The figure shows three views and two pictorial views of one solid part (mm, origin at its lowest corner). Answer the questions. Coordinates: 2 decimals unless noted, no trailing zeros. Order: outer loops, then holes, each group sorted by start corner. A loop starts at its lowest first (then second) coordinate and runs counter-clockwise, first axis right, second up. Notation, with made-up numbers: (-30, 33) -> (15, 33) arc R14 ccw to (15, 54) -> close; hole circle Ø2 at (65, 24.25). An arc over 180 degrees is marked (long way). Write item = value, one per line. Start each with the question number.
Q1. Straight lines are drawn through the part: L1, parallel to X at y = 309.5, z = 9.25; L2, parallel to Y at x = 487.5, z = 4; L3, parallel to X at y = 117, z = 6.5. For each, find the intervals that lie inside material, in ascending order. Write a range as from..to.
Q2. The part is cut by section D-D, the plane z = 14.75. Count the separate pieces of the cut face and the enclosed holes in it, plus the area to 3 significant figures.
Q3. The part is cut by section B-B, the plane y = 304.8. Determine the outline of the cut face in (x, z), plus the area to 3 significant figures.
Q4. A flat-ended cylindrical pin translates along its axis: pin 1 (5.5 mm diameter, centred on y = 216.5, z = 10.5, fed in from +X). Find the tip coordinate at first contact, or state that the pin passes through.
Q5. The part is cut by section A-A, the plane x = 44.45. Determine the outline of the cut face in (y, z).
Q6. For a pull along Z with two mould halves and no side action, classify the marked faces 1 and 2 as +Z half, -Z half, draft (parallel to the pull), parting line (faces both ways), or undercut.
Q7. The part is cut by section C-C, the plane x = 469. Determine the outline of the cut face in (y, z), plus the area to 3 significant figures.
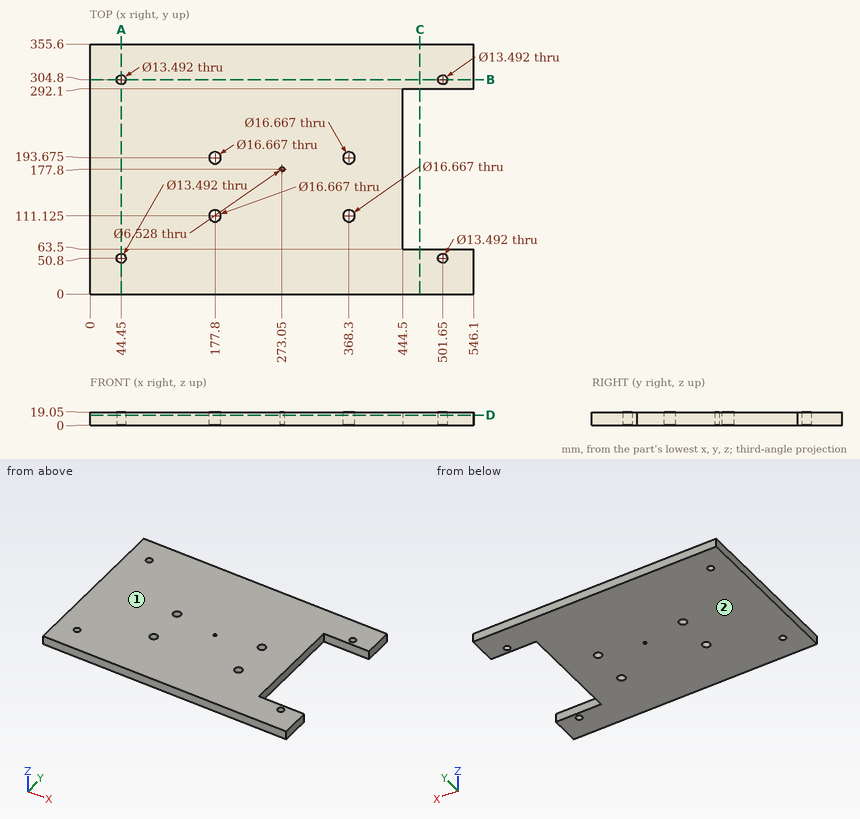
Model answer:
q1.L1 = 0..39.61, 49.29..496.81, 506.49..546.1
q1.L2 = 0..63.5, 292.1..355.6
q1.L3 = 0..171.89, 183.71..362.39, 374.21..444.5
q2.separate_pieces = 1
q2.enclosed_holes = 9
q2.area = 169,000 mm2
q3.outline = (0, 0) -> (37.7, 0) -> (37.7, 19.05) -> (0, 19.05) -> close; (51.2, 0) -> (494.9, 0) -> (494.9, 19.05) -> (51.2, 19.05) -> close; (508.4, 0) -> (546.1, 0) -> (546.1, 19.05) -> (508.4, 19.05) -> close
q3.area = 9,890 mm2
q4.pin_1 = 444.5
q5.outline = (0, 0) -> (44.05, 0) -> (44.05, 19.05) -> (0, 19.05) -> close; (57.55, 0) -> (298.05, 0) -> (298.05, 19.05) -> (57.55, 19.05) -> close; (311.55, 0) -> (355.6, 0) -> (355.6, 19.05) -> (311.55, 19.05) -> close
q6.face_1 = +Z half
q6.face_2 = -Z half
q7.outline = (0, 0) -> (63.5, 0) -> (63.5, 19.05) -> (0, 19.05) -> close; (292.1, 0) -> (355.6, 0) -> (355.6, 19.05) -> (292.1, 19.05) -> close
q7.area = 2,420 mm2
